from build123d import *

# Parameters (mm, degrees)
SKETCH1_R               = 5
BOSS_EXTRUDE1_DEPTH     = 5
SKETCH2_R               = 5.5
BOSS_EXTRUDE2_DEPTH     = 0.4
CUT_EXTRUDE1_DEPTH      = 6.4
SKETCH5_R               = 6
CUT_EXTRUDE2_DEPTH      = 6.5
CUT_EXTRUDE2_DEPTH_BACK = 6.5
CHAMFER4_SIZE           = 0.3
CHAMFER4_SIZE2          = 0.24293521


with BuildPart() as part:
    # Sketch1 → Boss-Extrude1 (new body)
    with BuildSketch(Plane(origin=(0, 0, 0), x_dir=(1, 0, 0), z_dir=(0, 1, 0))):
        Circle(SKETCH1_R)
    extrude(amount=BOSS_EXTRUDE1_DEPTH)

    # Sketch2 → Boss-Extrude2 (add)
    with BuildSketch(Plane(origin=(0, 5, 0), x_dir=(1, 0, 0), z_dir=(0, 1, 0))):
        Circle(SKETCH2_R)
    extrude(amount=BOSS_EXTRUDE2_DEPTH)

    # Sketch4 → Cut-Extrude1 (cut, through all)
    with BuildSketch(Plane(origin=(0, 5.4, 0), x_dir=(1, 0, 0), z_dir=(0, 1, 0))):
        with BuildLine():
            Line((2.295250379, 2.551364647), (2.295250379, -2.448635353))
            ThreePointArc((2.295250379, -2.448635353), (0, -4.743885732), (-2.295250379, -2.448635353))
            Line((-2.295250379, -2.448635353), (-2.295250379, 2.551364647))
            ThreePointArc((-2.295250379, 2.551364647), (0, 4.846615026), (2.295250379, 2.551364647))
        make_face()
    extrude(amount=-CUT_EXTRUDE1_DEPTH, mode=Mode.SUBTRACT)

    # Sketch5 → Cut-Extrude2 (cut, two sides)
    with BuildSketch(Plane(origin=(0, 0, 0), x_dir=(0, 0, -1), z_dir=(1, 0, 0))) as cut_extrude2_sk:
        with Locations((0, -1)):
            Circle(SKETCH5_R)
    extrude(amount=CUT_EXTRUDE2_DEPTH, mode=Mode.SUBTRACT)
    extrude(cut_extrude2_sk.sketch, amount=-CUT_EXTRUDE2_DEPTH_BACK, mode=Mode.SUBTRACT)

    # Chamfer4
    chamfer4_edges = [part.edges().sort_by_distance(p)[0] for p in [
        (0, 5.4, -4.846615026),
        (-2.295250379, 5.4, -0.051364647),
        (0, 5.4, 4.743885732),
        (2.295250379, 5.4, -0.051364647),
    ]]
    chamfer4_side = [part.faces().sort_by_distance(p)[0] for p in [
        (-5.344436508, 5.4, 0),
    ]]
    chamfer(chamfer4_edges, length=CHAMFER4_SIZE, length2=CHAMFER4_SIZE2, reference=chamfer4_side[0])


solid = part.part
The model under review builds one solid part; all positions refer to its coordinate system, in mm. A direction names the side the tool comes from. Give positions to 0.01 mm unless a question says otherwise; leave off trailing zeros. Loops run counter-clockwise (first coordinate to the right, second up) from the corner with the lowest first, then second, coordinate; pieces in that order, holes last. Notation, with made-up numbers: (-12, 35.25) -> (10, 35.25) arc R20 cw to (10, 41.25) -> close; hole circle Ø10 at (18.25, 1). An arc over 180 degrees is marked (long way). Answer as a JSON object with one key per item and string values. Group by question number.
Q1. Take a section at B-B (y = 3.4). Write out the cut boundary in (x, z).
Q2. Insertion check: pin 1 (1 mm diameter, centred on y = 4, z = 4, fed in from -X). The pin has a flat end and moves straight along its axis. Give the tip position at first contact, or say it passes through.
Q3. Take a section at D-D (x = -3.5). Write out the cut boundary in (y, z), plus the area to 3 significant figures.
Q4. Take a section at A-A (z = -0.75). Write out the cut boundary in (x, y).
Q5. Wall thickness on line 1 along X through (y, z) = (5.05, 1.5); line 2 along Z through (x, y) = (-1, 3.45); line 3 along X through (y, z) = (3.8, 3.75): over which ranges is each line inside the solid? List them lowest first.
Q6. Take a section at C-C (x = 4.75). Write out the cut boundary in (y, z).
Q7. Tool access review of faces 1 (the flat face through (1.6, 5, 4.9)), 2 (the cylindrical face through (0.05, 4.209, 4.743)), 3 (the cylindrical face through (0, 4, -5)), 4 (the conical face through (-0.054, 5.277, -4.994)): name each direction out of +Z, -Z, +X, -X, +Y, -Y from which nothing blocks a thin tool from reaching the whole face with its end or side.
Answer below:
{
 "1": {"outline": "(-2.89, -4.08) arc R5 ccw to (2.89, -4.08) -> (1.71, -4.08) arc R2.3 cw to (-1.71, -4.08) -> close; (-2.89, 4.08) -> (-1.62, 4.08) arc R2.3 cw to (1.62, 4.08) -> (2.89, 4.08) arc R5 ccw to start"},
 "2": {"pin 1": "stops at x = -3.57"},
 "3": {"outline": "(3.82, -3.57) -> (5, -3.57) -> (5, -4.24) -> (5.4, -4.24) -> (5.4, 4.24) -> (5, 4.24) -> (5, 3.57) -> (3.82, 3.57) arc R6 cw to start", "area": "6.08 mm2"},
 "4": {"outline": "(-5.45, 5) -> (-4.94, 5) -> (-4.94, 4.95) -> (-2.3, 4.95) -> (-2.3, 5.16) -> (-2.6, 5.4) -> (-5.45, 5.4) -> close; (2.3, 4.95) -> (4.94, 4.95) -> (4.94, 5) -> (5.45, 5) -> (5.45, 5.4) -> (2.6, 5.4) -> (2.3, 5.16) -> close"},
 "5": {"line 1": "x = -5.29 to -2.3, 2.3 to 5.29", "line 2": "z = -4.9 to -4.62, 4.51 to 4.9", "line 3": "x = -3.31 to -1.89, 1.89 to 3.31"},
 "6": {"outline": "(4.79, -1.56) -> (5, -1.56) -> (5, -2.77) -> (5.4, -2.77) -> (5.4, 2.77) -> (5, 2.77) -> (5, 1.56) -> (4.79, 1.56) arc R6 cw to start"},
 "7": {"face 1": "-Y", "face 2": "+Y, -Y", "face 3": "-Z, -Y", "face 4": "+Y"}
}
